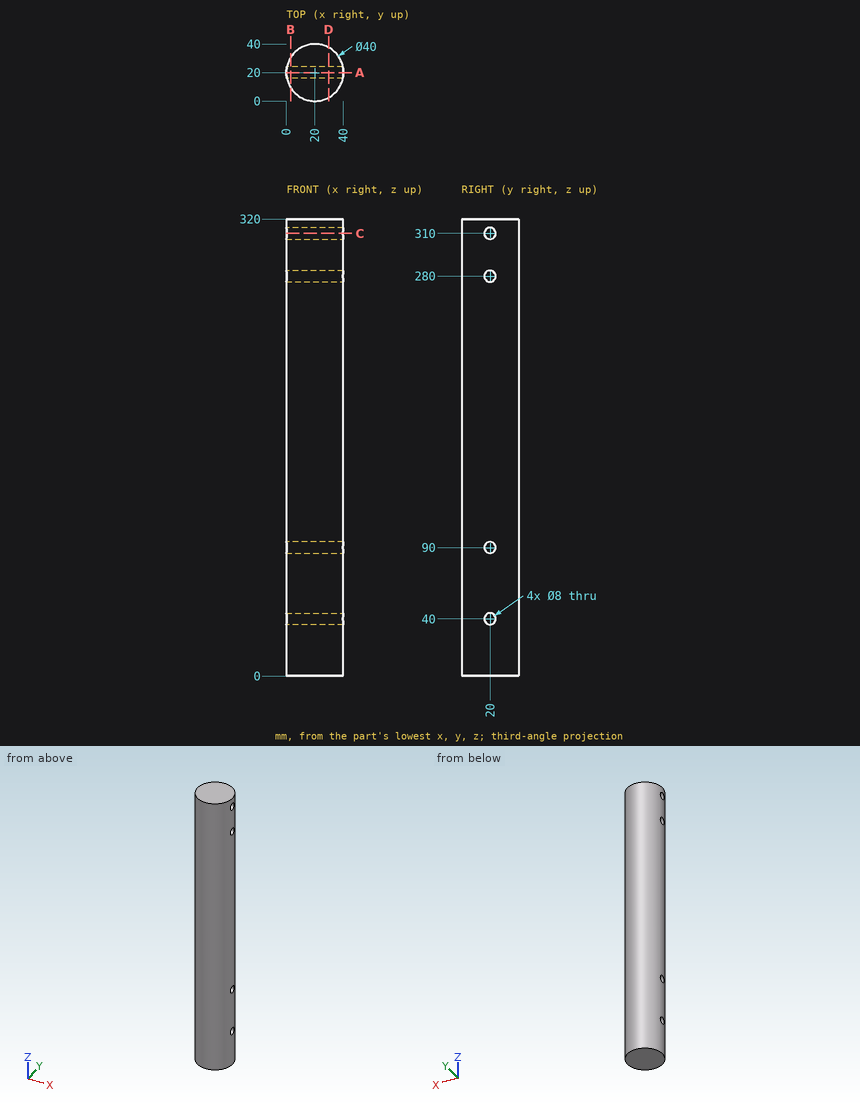
Can you work these out from the drawing? Everything is in mm from the part's minimum corner. Coordinates: 2 decimals unless noted, no trailing zeros. Loops run counter-clockwise (first coordinate to the right, second up) from the corner with the lowest first, then second, coordinate; pieces in that order, holes last. Notation, with made-up numbers: M 67.25,21.25 L 119.25,21.25 A18 ccw 119.25,54.25 Z; hole C -4.75,58 d3. An arc over 180 degrees is marked long. Put each result on its own line as item: value. Start each with the question number.
(1) Suppose I cut it at B-B on x = 3. Please give me the cut outline in (y, z), then the cut area to 3 significant figures.
(2) I need wall thicknesses on line 1 (Y direction, x = 25, z = 90); line 2 (Y direction, x = 20.5, z = 87); line 3 (Y direction, x = 19.5, z = 297). Which ranges of each line are inside material? Lowest first, please. Write a range as from..to.
(3) Suppose I cut it at A-A on y = 20. Please give me the cut outline in (x, z).
(4) Suppose I cut it at C-C on z = 310. Please give me the cut outline in (x, y).
(5) Will these pins go through, and if not, where does the flat tip stop? P1, Ø12, axis at x = 16.5, z = 132.5, coming from the -Y side; P2, Ø12, axis at y = 33.5, z = 228, coming from the -X side; P3, Ø12, axis at x = 21, z = 265, coming from the +Y side.
(6) Suppose I cut it at D-D on x = 29.5. Please give me the cut outline in (y, z), then the cut area to 3 significant figures.
Solutions:
1. outline: M 9.46,0 L 30.54,0 L 30.54,320 L 9.46,320 Z; hole C 20,40 d8; hole C 20,90 d8; hole C 20,280 d8; hole C 20,310 d8
1. area: 6,540 mm2
2. line 1: y = 0.64..16, 24..39.36
2. line 2: y = 0.01..17.35, 22.65..39.99
2. line 3: y = 0.01..39.99
3. outline: M 0,0 L 40,0 L 40,36 L 0,36 Z; M 0,44 L 40,44 L 40,86 L 0,86 Z; M 0,94 L 40,94 L 40,276 L 0,276 Z; M 0,284 L 40,284 L 40,306 L 0,306 Z; M 0,314 L 40,314 L 40,320 L 0,320 Z
4. outline: M 0.4,16 A20 ccw 39.6,16 Z; M 0.4,24 L 39.6,24 A20 ccw Z
5. P1: stops at y = 0
5. P2: stops at x = 1.46
5. P3: stops at y = 40
6. outline: M 2.4,0 L 37.6,0 L 37.6,320 L 2.4,320 Z; hole C 20,40 d8; hole C 20,90 d8; hole C 20,280 d8; hole C 20,310 d8
6. area: 11,100 mm2
